Can you work these out from the model? Positions are in its coordinate system, mm. Round coordinates to 2 decimals unless told otherwise and drop trailing zeros. Write item = value, one per line. Start each with the question number.
1) I'm going to push flat-ended pins straight in: pin 1 (1.5 mm diameter, centred on y = -14.5, z = 0.5, fed in from +X); pin 2 (2.5 mm diameter, centred on x = -16.63, y = 14.41, fed in from +Z); pin 3 (2 mm diameter, centred on y = 5, z = 1, fed in from -X); pin 4 (1.5 mm diameter, centred on y = -13.5, z = 3.5, fed in from -X). Where does each tip first touch, or does it pass through?
2) If I drill on line 1 (Y direction, x = -14, z = 2); line 2 (Y direction, x = -9.5, z = 3.7); line 3 (Y direction, x = -4, z = 2), over which ranges is the centre line in solid material (lowest first)?
3) Imagine slicing it at A-A, the plane x = 0. State how many separate pieces and enclosed holes the cut face has, then the cut area to 3 significant figures.
from build123d import *

# Parameters (mm, degrees)
SKETCH1_R           = 5
BOSS_EXTRUDE1_DEPTH = 4
SKETCH2_R           = 1.5
CUT_EXTRUDE1_DEPTH  = 40.824615503
CIRPATTERN1_COUNT   = 22


with BuildPart() as part:
    # Sketch1 → Boss-Extrude1 (new body)
    with BuildSketch(Plane.XY):
        with BuildLine():
            ThreePointArc((-1.998627787, 26.925925926), (0, -27), (1.998627787, 26.925925926))
            ThreePointArc((1.998627787, 26.925925926), (0, 29), (-1.998627787, 26.925925926))
        make_face()
        Circle(SKETCH1_R, mode=Mode.SUBTRACT)
    extrude(amount=BOSS_EXTRUDE1_DEPTH)

    # Sketch2 → Cut-Extrude1 (cut, through all)
    with BuildSketch(Plane.XY.offset(4)):
        with Locations((0, 13)):
            Circle(SKETCH2_R)
        with Locations((0, 17.5)):
            Circle(SKETCH2_R)
        with Locations((0, 22)):
            Circle(SKETCH2_R)
    cut_extrude1 = extrude(amount=-CUT_EXTRUDE1_DEPTH, mode=Mode.SUBTRACT)

    # CirPattern1: Cut-Extrude1 ×22 about axis
    cirpattern1_axis = Axis((0, 0, 0), (0, 0, 1))
    for i in range(1, CIRPATTERN1_COUNT):
        add(cut_extrude1.rotate(cirpattern1_axis, i * 360 / CIRPATTERN1_COUNT), mode=Mode.SUBTRACT)


solid = part.part
Reported:
q1.pin_1 = 23.24
q1.pin_2 = through
q1.pin_3 = -26.7
q1.pin_4 = -23.8
q2.line_1 = -23.09 to -12.74, -10.18 to -2.83, -0.87 to 0.87, 2.83 to 10.18, 12.74 to 23.09
q2.line_2 = -25.27 to -16.22, -13.22 to -9.98, -7.05 to 7.05, 9.98 to 13.22, 16.22 to 25.27
q2.line_3 = -26.7 to -17.97, -15.61 to -13.93, -11.01 to -3, 3 to 11.01, 13.93 to 15.61, 17.97 to 26.7
q3.separate_pieces = 8
q3.enclosed_holes = 0
q3.area = 112 mm²
